```python
from build123d import *

# Parameters (mm, degrees)
F0_R     = 7
F1_DEPTH = 22
F2_R     = 7
F3_DEPTH = 19
F2_R_2   = 5.5
F4_DEPTH = 44.001
F7_DEPTH = 24


with BuildPart() as f1:
    # F0 (on Front) → F1 (new body, symmetric)
    with BuildSketch(Plane.XZ):
        with BuildLine():
            Line((-7, 18), (-14, 11))
            Line((-14, 11), (-14, -7))
            Line((-14, -7), (-7, -14))
            Line((-7, -14), (25.575539, -14))
            ThreePointArc((25.575539, -14), (28.840775, -15.213414), (30.521178, -18.264706))
            ThreePointArc((30.521178, -18.264706), (32.858008, -26.115672), (37.29698, -33))
            Line((37.29698, -33), (43, -33))
            Line((43, -33), (72, 1))
            Line((72, 1), (72, 20))
            Line((72, 20), (67, 25))
            Line((67, 25), (43, 25))
            ThreePointArc((43, 25), (34.561099, 15.982044), (22.361381, 14.057085))
            Line((22.361381, 14.057085), (0, 18))
            Line((0, 18), (-7, 18))
        make_face()
        Circle(F0_R, mode=Mode.SUBTRACT)
    extrude(amount=F1_DEPTH, both=True)

    # F2 (on face) → F3 (cut)
    with BuildSketch(Plane.XZ.offset(22)):
        Polygon((20, -14), (20, 14.47346), (0, 18), (-7, 18), (-14, 11), (-14, -7), (-7, -14), align=None)
        Circle(F2_R, mode=Mode.SUBTRACT)
        with BuildLine():
            Line((59.205882, -14), (25.575539, -14))
            ThreePointArc((25.575539, -14), (28.840775, -15.213414), (30.521178, -18.264706))
            ThreePointArc((30.521178, -18.264706), (32.858008, -26.115672), (37.29698, -33))
            Line((37.29698, -33), (43, -33))
            Line((43, -33), (59.205882, -14))
        make_face()
    extrude(amount=-F3_DEPTH, mode=Mode.SUBTRACT)

    # F2 (on face) → F4 (cut, through all)
    with BuildSketch(Plane.XZ.offset(22)):
        with Locations((58, 11)):
            Circle(F2_R_2)
    extrude(amount=-F4_DEPTH, mode=Mode.SUBTRACT)

    # F6 (on offset) → F7 (cut)
    with BuildSketch(Plane.XZ.offset(-10)):
        with BuildLine():
            Line((72, 25), (31.167462, 25))
            ThreePointArc((31.167462, 25), (40.759308, 2.149677), (61.764706, -11))
            Line((61.764706, -11), (72, 0))
            Line((72, 0), (72, 25))
        make_face()
    extrude(amount=F7_DEPTH, mode=Mode.SUBTRACT)


solid = f1.part
```
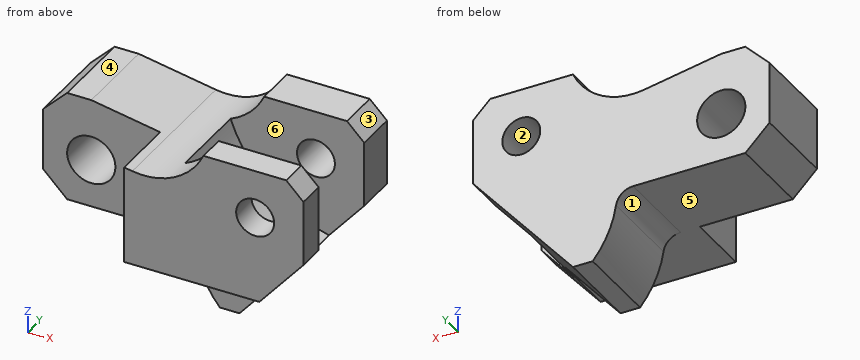
Work out the finished part from the listing and answer in its coordinate system (mm). Face numbers are marked on the shaded views. A direction names the side the tool comes from. Coordinates: 2 decimals unless noted, no trailing zeros. Write each loop counter-clockwise with the first axis right and the second up, starting at its lowest first coordinate (ties: lowest second). Pieces come first, ordered by that corner, then holes. Notation, with made-up numbers: (-33.75, 57.5) - (13.25, 57.5) arc R12 ccw to (13.25, 61.5) - close; hole circle Ø7 at (13, 15). An arc over 180 degrees is marked (long way). Answer as a JSON object with one key per item and string values.
Q1. For a pull along X with two mould halves and no side action, classify the marked faces 1, 2 and 3 as pulls with the +X half, pulls with the -X half, needs draft (parallel to the pull), parting line crosses it, or undercut.
Results list:
{"face 1": "pulls with the -X half", "face 2": "undercut", "face 3": "pulls with the +X half"}
Q2. Consider L1, parallel to Y at x = 54.5, z = 22; L2, parallel to Z at x = 58, y = -19.75; L3, parallel to Z at x = 0, y = 11.5. Determine where each line is inside the solid, lowest interval first. Write a range as from..to.
Results list:
{"L1": "y = -22..-14, 10..22", "L2": "z = -14..5.5, 16.5..25", "L3": "z = -14..-7, 7..18"}
Q3. Find section D-D (y = 13.5). Write down the section's boundary in (x, z), plus the area to 3 significant figures.
Results list:
{"outline": "(-14, -7) - (-7, -14) - (25.58, -14) arc R5 cw to (30.52, -18.26) arc R29 ccw to (37.3, -33) - (43, -33) - (72, 1) - (72, 20) - (67, 25) - (43, 25) arc R19 cw to (22.36, 14.06) - (0, 18) - (-7, 18) - (-14, 11) - close; hole circle Ø14 at (0, 0); hole circle Ø11 at (58, 11)", "area": "2,830 mm^2"}
Q4. Find section C-C (x = -2.5). Write down the section's boundary in (y, z).
Results list:
{"outline": "(-3, -14) - (22, -14) - (22, -6.54) - (-3, -6.54) - close; (-3, 6.54) - (22, 6.54) - (22, 18) - (-3, 18) - close"}
Q5. Find section A-A (y = -18). Write down the section's boundary in (x, z).
Results list:
{"outline": "(20, -14) - (59.21, -14) - (72, 1) - (72, 20) - (67, 25) - (43, 25) arc R19 cw to (22.36, 14.06) - (20, 14.47) - close; hole circle Ø11 at (58, 11)"}
Q6. Find section B-B (z = 2). Write down the section's boundary in (x, y), plus the area to 3 significant figures.
Results list:
{"outline": "(-14, -3) - (-6.71, -3) - (-6.71, 22) - (-14, 22) - close; (6.71, -3) - (20, -3) - (20, -22) - (72, -22) - (72, -14) - (40.89, -14) - (40.89, 10) - (72, 10) - (72, 22) - (6.71, 22) - close", "area": "2,060 mm^2"}
Q7. Which of the six approach directions +Z, -Z, +X, -X, +Y, -Y give full straight-line access (tool end or side, diameter ignored) to the marked faces 4, 5 and 6?
Results list:
{"face 4": "+Z, -X, +Y, -Y", "face 5": "-Z, -X, -Y", "face 6": "+Z, +X"}
Q8. Given pin 1 Ø4 at (x, z) = (35, -19) entering from -Y; pin 2 Ø21 at (y, z) = (-15, 1) entering from -X; pin 3 Ø12.5 at (x, z) = (58, 11) entering from +Y; pin 4 Ø10 at (y, z) = (11, -22) entering from -X, each flat-ended and moving along its own axis, determine where each tip first touches the part or whether it passes through.
Results list:
{"pin 1": "stops at y = -3", "pin 2": "stops at x = 20", "pin 3": "stops at y = 22", "pin 4": "stops at x = 30.16"}
